The listing builds one solid part. Answer for the finished solid, in the listing's coordinates (mm). Face numbers are marked on the shaded views. A direction names the side the tool comes from. Coordinates: 2 decimals unless noted, no trailing zeros. Order: outer loops, then holes, each group sorted by start corner. A loop starts at its lowest first (then second) coordinate and runs counter-clockwise, first axis right, second up. Notation, with made-up numbers: (62, -12) -> (77, -12) arc R29 cw to (77, 11) -> close; hole circle Ø10 at (81, 58). An arc over 180 degrees is marked (long way). Write each question's results on one line, items separated by ' | '. Start each with the question number.
(1) Given pin 1 (1 mm diameter, centred on x = -6, y = -30, fed in from -Z); pin 2 (1.1 mm diameter, centred on y = -0.5, z = -1, fed in from -X); pin 3 (1.5 mm diameter, centred on x = -13, z = -23, fed in from -Y), each flat-ended and moving along its own axis, determine where each tip first touches the part or whether it passes through.
(2) The part is cut by section B-B, the plane z = 25. Give the vertices of the cut face in (x, y).
(3) The part is cut by section A-A, the plane x = -26. Give the vertices of the cut face in (y, z).
(4) A tool of negligible diameter and unlimited length cuts with its end or side. For the marked faces 1 and 2, from which of +Z, -Z, +X, -X, +Y, -Y can it reach the whole face along a straight path? Write none if from no direction.
(5) The part is cut by section C-C, the plane y = -8. Give the vertices of the cut face in (x, z).
(6) Determine the mould class of the marked faces 3, 4, 5 and 6 for opening direction Z: +Z half, -Z half, draft (parallel to the pull), parting line (faces both ways), or undercut.
(7) Straight lines are drawn through the part: L1, parallel to Y at x = -13, z = -3.5; L2, parallel to X at y = -35, z = 0.5; L3, parallel to Y at x = -20, z = 23. For each, find the intervals that lie inside material, in ascending order.
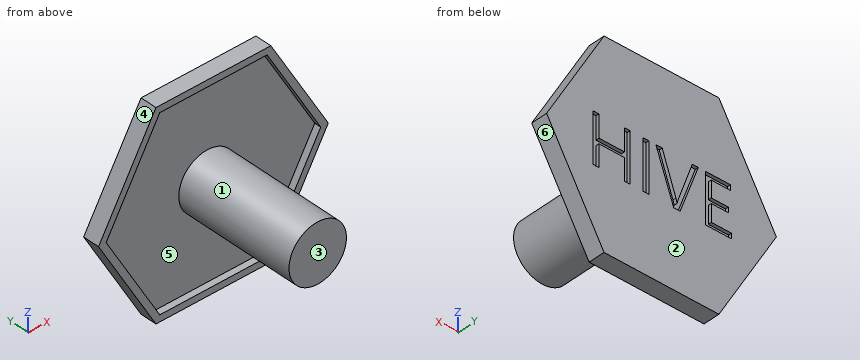
Autodesk Inventor part; units mm, degrees
ref_plane "YZ Plane" through (0, 0, 0) normal (1, 0, 0) x (0, 1, 0)
ref_plane "XZ Plane" through (0, 0, 0) normal (0, 1, 0) x (-1, 0, 0)
ref_plane "XY Plane" through (0, 0, 0) normal (0, 0, 1) x (1, 0, 0)
sketch "Sketch1" plane through (0, 0, 0) normal (0, 1, 0) x (-1, 0, 0)
  circle A0 centre (0, 0) radius 35
  line L0 (17.5, -30.3109) -> (-17.5, -30.3109)
  line L1 (-17.5, -30.3109) -> (-35, 0)
  line L2 (-35, 0) -> (-17.5, 30.3109)
  line L3 (-17.5, 30.3109) -> (17.5, 30.3109)
  line L4 (17.5, 30.3109) -> (35, 0)
  line L5 (35, 0) -> (17.5, -30.3109)
  line L6 (16.3453, -28.3109) -> (-16.3453, -28.3109)
  line L7 (-16.3453, -28.3109) -> (-32.6906, 0)
  line L8 (-32.6906, 0) -> (-16.3453, 28.3109)
  line L9 (-16.3453, 28.3109) -> (16.3453, 28.3109)
  line L10 (16.3453, 28.3109) -> (32.6906, 0)
  line L11 (32.6906, 0) -> (16.3453, -28.3109)
  line L12 (0, 0) -> (-17.5, -30.3109)
  circle A1 centre (0, 0) radius 8.75
  line L13 (-22.7839, 7.707) -> (22.7839, 7.707) construction
  line L14 (22.7839, 7.707) -> (22.7839, -7.707) construction
  line L15 (22.7839, -7.707) -> (-22.7839, -7.707) construction
  line L16 (-22.7839, -7.707) -> (-22.7839, 7.707) construction
  line L17 (0, 0) -> (0, -28.3109) construction
  line L18 (1.5082, 8.619) -> (10.7506, 8.619) construction
  line L19 (-22.7839, 0) -> (22.7839, 0) construction
  line L20 (0, 7.707) -> (0, -7.707) construction
  line L21 (-20.822, 7.707) -> (-19.0548, 7.707)
  line L22 (-19.0548, 7.707) -> (-19.0548, 0.9167)
  line L23 (-19.0548, 0.9167) -> (-11.2904, 0.9167)
  line L24 (-11.2904, 0.9167) -> (-11.2904, 7.707)
  line L25 (-11.2904, 7.707) -> (-9.5372, 7.707)
  line L26 (-9.5372, 7.707) -> (-9.5372, -7.293)
  line L27 (-9.5372, -7.293) -> (-11.2904, -7.293)
  line L28 (-11.2904, -7.293) -> (-11.2904, -0.6557)
  line L29 (-11.2904, -0.6557) -> (-19.0548, -0.6557)
  line L30 (-19.0548, -0.6557) -> (-19.0548, -7.293)
  line L31 (-19.0548, -7.293) -> (-20.822, -7.293)
  line L32 (-20.822, -7.293) -> (-20.822, 7.707)
  line L33 (-5.6133, 7.707) -> (-3.8461, 7.707)
  line L34 (-3.8461, 7.707) -> (-3.8461, -7.293)
  line L35 (-3.8461, -7.293) -> (-5.6133, -7.293)
  line L36 (-5.6133, -7.293) -> (-5.6133, 7.707)
  line L37 (-1.7032, 7.707) -> (0.217, 7.707)
  line L38 (0.217, 7.707) -> (4.4053, -4.2456)
  spline S0 degree 2 poles (4.4053, -4.2456) (4.6279, -4.8301) (4.7253, -5.5815) knots 0 0 0 1 1 1
  line L39 (4.7253, -5.5815) -> (4.7671, -5.5815)
  spline S1 degree 2 poles (4.7671, -5.5815) (4.8506, -5.011) (5.1149, -4.2178) knots 0 0 0 1 1 1
  line L40 (5.1149, -4.2178) -> (9.3867, 7.707)
  line L41 (9.3867, 7.707) -> (11.2235, 7.707)
  line L42 (11.2235, 7.707) -> (5.6715, -7.3069)
  line L43 (5.6715, -7.3069) -> (3.7374, -7.3069)
  line L44 (3.7374, -7.3069) -> (-1.7032, 7.707)
  line L45 (13.3942, 7.707) -> (21.0194, 7.707)
  line L46 (21.0194, 7.707) -> (21.0194, 6.1208)
  line L47 (21.0194, 6.1208) -> (15.1613, 6.1208)
  line L48 (15.1613, 6.1208) -> (15.1613, 1.1254)
  line L49 (15.1613, 1.1254) -> (20.3654, 1.1254)
  line L50 (20.3654, 1.1254) -> (20.3654, -0.4469)
  line L51 (20.3654, -0.4469) -> (15.1613, -0.4469)
  line L52 (15.1613, -0.4469) -> (15.1613, -5.7067)
  line L53 (15.1613, -5.7067) -> (21.3534, -5.7067)
  line L54 (21.3534, -5.7067) -> (21.3534, -7.293)
  line L55 (21.3534, -7.293) -> (13.3942, -7.293)
  line L56 (13.3942, -7.293) -> (13.3942, 7.707)
  dimension "d0" = 70
  dimension "d2" = 17.5
  dimension "d1" = 2
extrude "Extrusion1" add sketch "Sketch1" against normal blind 3 contours L6 L7 L8 L9 L10 L11 | L35 L36 A1 | A1 L36 L33 | A1 L42 L43 | L40 L41 L42 A1 | L21 L22 L23 L24 L25 L26 L27 L28 L29 L30 L31 L32 | L45 L46 L47 L48 L49 L50 L51 L52 L53 L54 L55 L56
extrude "Extrusion3" add sketch "Sketch1" against normal blind 5 contours L5 L0 L1 L2 L3 L4
extrude "Extrusion4" add sketch "Sketch1" against normal blind 40 contours L34 L35 L12 | L12 L35 A1 L36 L33 L34 | L34 L33 A1 L40 S1 L39 S0 L38 L37 L44 L43 L12 L35 | L12 A1 L35 | L43 L44 L37 L38 S0 L39 S1 L40 A1 L42 | A1 L36 | L42 A1
extrude "Extrusion6" cut sketch "Sketch1" against normal blind 1 contours L34 L35 L12 | L12 L35 A1 L36 L33 L34 | L35 L36 A1 | A1 L36 L33 | L43 L44 L37 L38 S0 L39 S1 L40 A1 L42 | A1 L42 L43 | L40 L41 L42 A1 | L21 L22 L23 L24 L25 L26 L27 L28 L29 L30 L31 L32 | L45 L46 L47 L48 L49 L50 L51 L52 L53 L54 L55 L56
equation "\"d0\" = diam"
equation "\"d2\" = 0.25 * diam"
equation "\"d3\" = thickness"
equation "\"d9\" = 8 * d5"
equation "\"thickness\" = 3"
properties part number "stand"
Established:
1) pin 1: stops at z = -6.81 | pin 2: stops at x = -34.74 | pin 3: stops at y = -3
2) outline: (-20.57, -5) -> (-18.26, -5) -> (-18.26, -3) -> (18.26, -3) -> (18.26, -5) -> (20.57, -5) -> (20.57, 0) -> (-20.57, 0) -> close
3) outline: (-5, -15.59) -> (0, -15.59) -> (0, 15.59) -> (-5, 15.59) -> (-5, 11.59) -> (-3, 11.59) -> (-3, -11.59) -> (-5, -11.59) -> close
4) face 1: -Y | face 2: +Z, -Z, +X, -X, +Y
5) outline: circle Ø17.5 at (0, 0)
6) face 3: draft | face 4: +Z half | face 5: undercut | face 6: -Z half
7) L1: y = -3 to 0 | L2: x = -8.74 to 8.74 | L3: y = -5 to 0
